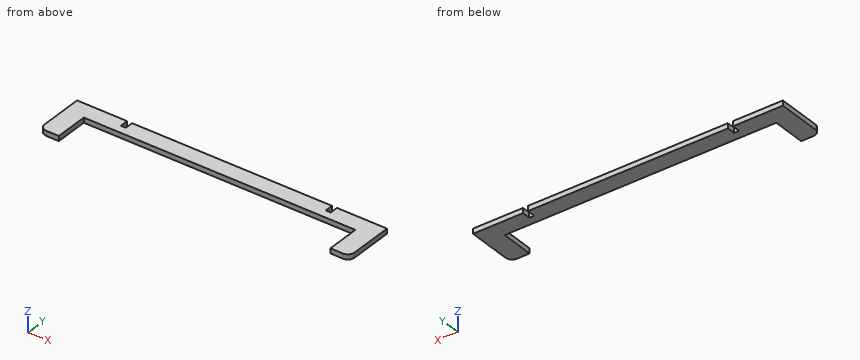
```python
from build123d import *

# Parameters (mm, degrees)
BOSS_EXTRUDE1_DEPTH = 3
SKETCH2_W           = 163
SKETCH2_H           = 40
CUT_EXTRUDE1_DEPTH  = 3
FILLET1_R           = 4


with BuildPart() as part:
    # Sketch1 → Boss-Extrude1 (new body)
    with BuildSketch(Plane.XY):
        Polygon((-93, 15), (-63, 15), (-63, 10), (-60, 10), (-60, 15), (60, 15), (60, 10), (63, 10), (63, 15), (93, 15), (93, -15), (-93, -15), align=None)
    extrude(amount=BOSS_EXTRUDE1_DEPTH)

    # Sketch2 → Cut-Extrude1 (cut)
    with BuildSketch(Plane.XY.offset(3)):
        with Locations((0, -15)):
            Rectangle(SKETCH2_W, SKETCH2_H)
    extrude(amount=-CUT_EXTRUDE1_DEPTH, mode=Mode.SUBTRACT)

    # Fillet1
    fillet1_edges = [part.edges().sort_by_distance(p)[0] for p in [
        (93, -15, 1.5),
        (-93, -15, 1.5),
    ]]
    fillet(fillet1_edges, radius=FILLET1_R)


solid = part.part
```
For this review, take the finished solid that the model builds, in its own axes (mm). Coordinates: 2 decimals unless noted, no trailing zeros. Loops run counter-clockwise (first coordinate to the right, second up) from the corner with the lowest first, then second, coordinate; pieces in that order, holes last. Notation, with made-up numbers: (-13.5, 2) -> (25.5, 2) arc R14 cw to (25.5, 11) -> close; hole circle Ø9 at (-14.75, -33.5). An arc over 180 degrees is marked (long way). Return JSON: item names as keys, results as strings. Group by question number.
(1) For pin 1 Ø1 at (x, z) = (37, 2.5) entering from -Y; pin 2 Ø1.5 at (x, z) = (62, 2) entering from +Y, all flat-tipped, find the tip position at first contact; note any pin that passes through.
(2) Consider section C-C, the plane x = 25. Give the boundary of the cut face in (y, z), plus the area to 3 significant figures.
(3) Consider section A-A, the plane y = 0.25. Give the boundary of the cut face in (x, z).
(4) Consider section B-B, the plane z = 0.85. Give the boundary of the cut face in (x, y).
(5) To check wall thickness, follow L1, parallel to X at y = 12.75, z = 1.3; L2, parallel to X at y = 4.5, z = 2.2; L3, parallel to Y at x = -43, z = 1.5. State the ranges of each line that lie inside material, in increasing order.
Results below:
{
 "1": {"pin 1": "stops at y = 5", "pin 2": "stops at y = 10"},
 "2": {"outline": "(5, 0) -> (15, 0) -> (15, 3) -> (5, 3) -> close", "area": "30.0 mm2"},
 "3": {"outline": "(-93, 0) -> (-81.5, 0) -> (-81.5, 3) -> (-93, 3) -> close; (81.5, 0) -> (93, 0) -> (93, 3) -> (81.5, 3) -> close"},
 "4": {"outline": "(-93, -11) arc R4 ccw to (-89, -15) -> (-81.5, -15) -> (-81.5, 5) -> (81.5, 5) -> (81.5, -15) -> (89, -15) arc R4 ccw to (93, -11) -> (93, 15) -> (63, 15) -> (63, 10) -> (60, 10) -> (60, 15) -> (-60, 15) -> (-60, 10) -> (-63, 10) -> (-63, 15) -> (-93, 15) -> close"},
 "5": {"L1": "x = -93 to -63, -60 to 60, 63 to 93", "L2": "x = -93 to -81.5, 81.5 to 93", "L3": "y = 5 to 15"}
}
